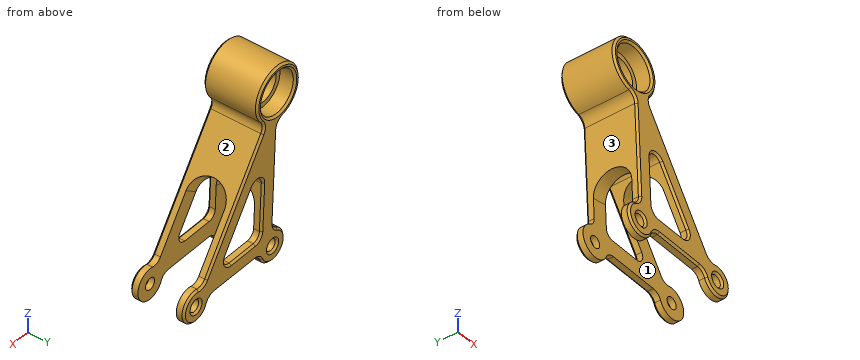
from build123d import *

# Parameters (mm, degrees)
SKETCH1_R                       = 14
BOSS_EXTRUDE1_DEPTH             = 14
SKETCH4_R                       = 11
CUT_EXTRUDE1_DEPTH              = 8
SKETCH5_R                       = 8.5
CUT_EXTRUDE2_DEPTH              = 21
BOSS_EXTRUDE2_REACH             = 16
BOSS_EXTRUDE2_DIRECTION_2_REACH = 16
SKETCH8_R                       = 3
CUT_EXTRUDE3_DEPTH              = 15
CUT_EXTRUDE3_DEPTH_BACK         = 15
FILLET1_R                       = 5
FILLET2_R                       = 4
CHAMFER1_SIZE                   = 1


with BuildPart() as part:
    # Sketch1 → Boss-Extrude1 (new body, symmetric)
    with BuildSketch(Plane(origin=(0, 0, 0), x_dir=(1, 0, 0), z_dir=(0, 1, 0))):
        Circle(SKETCH1_R)
    extrude(amount=BOSS_EXTRUDE1_DEPTH, both=True)

    # Sketch4 → Cut-Extrude1 (cut)
    with BuildSketch(Plane(origin=(0, 14, 0), x_dir=(1, 0, 0), z_dir=(0, 1, 0))):
        Circle(SKETCH4_R)
    cut_extrude1 = extrude(amount=-CUT_EXTRUDE1_DEPTH, mode=Mode.SUBTRACT)

    # Mirror1: Cut-Extrude1 across plane
    add(cut_extrude1.mirror(Plane.ZX), mode=Mode.SUBTRACT)

    # Sketch5 → Cut-Extrude2 (cut, through all)
    with BuildSketch(Plane(origin=(0, 6, 0), x_dir=(1, 0, 0), z_dir=(0, 1, 0))):
        Circle(SKETCH5_R)
    extrude(amount=-CUT_EXTRUDE2_DEPTH, mode=Mode.SUBTRACT)

    # Boss-Extrude2: up to this face of the body (flat: up to its plane)
    boss_extrude2_end = Plane(part.part.faces().sort_by_distance((-13.604020203, 14, 0))[0])
    # Sketch6 → Boss-Extrude2 (add, up to the picked face)
    with BuildSketch(Plane(origin=(0, 0, 0), x_dir=(1, 0, 0), z_dir=(0, 1, 0)), mode=Mode.PRIVATE) as boss_extrude2_sk1:
        with BuildLine():
            Line((0, 0), (49.796956955, 71.339071188))
            ThreePointArc((49.796956955, 71.339071188), (61.469373279, 81.598158377), (46.37598748, 77.89898578))
            Line((46.37598748, 77.89898578), (11.968376795, 77.89898578))
            ThreePointArc((11.968376795, 77.89898578), (-1.542698235, 83.697955691), (3.56136379, 69.909346213))
            Line((3.56136379, 69.909346213), (0, 0))
        make_face()
        Polygon((9.409062598, 27.456171423), (39.035506627, 69.89898578), (11.57120987, 69.89898578), align=None, mode=Mode.SUBTRACT)
    boss_extrude2_tool1 = split(extrude(boss_extrude2_sk1.sketch, amount=BOSS_EXTRUDE2_REACH, mode=Mode.PRIVATE), bisect_by=boss_extrude2_end, keep=Keep.BOTH, mode=Mode.PRIVATE)
    add(boss_extrude2_tool1.solids().sort_by_distance((2.865029, 0, -34.899434))[0])

    # Boss-Extrude2 direction 2: up to this face of the body (flat: up to its plane)
    boss_extrude2_direction_2_end = Plane(part.part.faces().sort_by_distance((-13.604020203, -14, 0))[0])
    # Sketch6 → Boss-Extrude2 direction 2 (add, up to the picked face)
    with BuildSketch(Plane(origin=(0, 0, 0), x_dir=(1, 0, 0), z_dir=(0, 1, 0)), mode=Mode.PRIVATE) as boss_extrude2_direction_2_sk1:
        with BuildLine():
            Line((0, 0), (49.796956955, 71.339071188))
            ThreePointArc((49.796956955, 71.339071188), (61.469373279, 81.598158377), (46.37598748, 77.89898578))
            Line((46.37598748, 77.89898578), (11.968376795, 77.89898578))
            ThreePointArc((11.968376795, 77.89898578), (-1.542698235, 83.697955691), (3.56136379, 69.909346213))
            Line((3.56136379, 69.909346213), (0, 0))
        make_face()
        Polygon((9.409062598, 27.456171423), (39.035506627, 69.89898578), (11.57120987, 69.89898578), align=None, mode=Mode.SUBTRACT)
    boss_extrude2_direction_2_tool1 = split(extrude(boss_extrude2_direction_2_sk1.sketch, amount=-BOSS_EXTRUDE2_DIRECTION_2_REACH, mode=Mode.PRIVATE), bisect_by=boss_extrude2_direction_2_end, keep=Keep.BOTH, mode=Mode.PRIVATE)
    add(boss_extrude2_direction_2_tool1.solids().sort_by_distance((2.865029, 0, -34.899434))[0])

    # Sketch7 → Cut-Revolve1 (revolve, cut)
    with BuildSketch(Plane.XY):
        Polygon((0, 14), (0, -14), (11, -14), (11, -6), (8.5, -6), (8.5, 6), (11, 6), (11, 14), align=None)
    revolve(axis=Axis((0, 14, 0), (0, -1, 0)), mode=Mode.SUBTRACT)

    # Sketch8 → Cut-Extrude3 (cut, two sides)
    with BuildSketch(Plane(origin=(0, 0, 0), x_dir=(1, 0, 0), z_dir=(0, 1, 0))) as cut_extrude3_sk:
        with Locations((3.968376795, 77.89898578)):
            Circle(SKETCH8_R)
        with Locations((54.37598748, 77.89898578)):
            Circle(SKETCH8_R)
    extrude(amount=CUT_EXTRUDE3_DEPTH, mode=Mode.SUBTRACT)
    extrude(cut_extrude3_sk.sketch, amount=-CUT_EXTRUDE3_DEPTH_BACK, mode=Mode.SUBTRACT)

    # Fillet1
    fillet1_edges = [part.edges().sort_by_distance(p)[0] for p in [
        (8.013303418, 0, -11.479850536),
        (0.712272758, 0, -13.981869243),
        (3.56136379, 0, -69.909346213),
        (11.968376795, 0, -77.89898578),
        (46.37598748, 0, -77.89898578),
        (49.796956955, 0, -71.339071188),
    ]]
    fillet(fillet1_edges, radius=FILLET1_R)

    # Fillet2
    fillet2_edges = [part.edges().sort_by_distance(p)[0] for p in [
        (11.57120987, 0, -69.89898578),
        (39.035506627, 0, -69.89898578),
        (9.409062598, 0, -27.456171423),
    ]]
    fillet(fillet2_edges, radius=FILLET2_R)

    # Sketch10 → Cut-Revolve2 (revolve, cut)
    with BuildSketch(Plane.ZY.offset(4.031623205)):
        with BuildLine():
            Line((-115.89898578, 10), (-55.89898578, 10))
            ThreePointArc((-55.89898578, 10), (-45.89898578, 0), (-55.89898578, -10))
            Line((-55.89898578, -10), (-115.89898578, -10))
            Line((-115.89898578, -10), (-115.89898578, 10))
        make_face()
    revolve(axis=Axis((-4.031623205, 14, 0.161756304), (0, -1, 0)), mode=Mode.SUBTRACT)

    # Chamfer1
    chamfer1_edges = [part.edges().sort_by_distance(p)[0] for p in [
        (45.149488461, -14, -78.738734309),
        (45.149488461, 14, -78.738734309),
        (13.194875814, -14, -78.738734309),
        (13.194875814, 14, -78.738734309),
        (26.019387345, 14, -51.252106195),
        (26.019387345, -14, -51.252106195),
        (23.368946304, 14, -69.89898578),
        (23.368946304, -14, -69.89898578),
        (10.748290369, 14, -53.74512796),
        (10.748290369, -14, -53.74512796),
        (34.9119591, -14, -67.748572079),
        (34.9119591, 14, -67.748572079),
        (12.617088893, -14, -68.798470735),
        (12.617088893, 14, -68.798470735),
        (12.81684933, -14, -37.400283889),
        (12.81684933, 14, -37.400283889),
        (-6.296166971, -14, 9.019882564),
        (-6.296166971, 14, 9.019882564),
        (0.968376795, -14, -77.89898578),
        (0.968376795, 14, -77.89898578),
        (51.37598748, -14, -77.89898578),
        (51.37598748, 14, -77.89898578),
        (28.999659343, 14, -41.544883239),
        (28.999659343, -14, -41.544883239),
        (-4.538605987, 14, 13.243906361),
        (-4.538605987, -14, 13.243906361),
        (2.14522062, -14, -42.110545238),
        (2.14522062, 14, -42.110545238),
        (-1.542698235, 14, -83.697955691),
        (-1.542698235, -14, -83.697955691),
        (61.469373279, 14, -81.598158377),
        (61.469373279, -14, -81.598158377),
        (29.172182137, 14, -77.89898578),
        (29.172182137, -14, -77.89898578),
        (9.596412617, -14, -11.95458808),
        (9.596412617, 14, -11.95458808),
        (-0.246894433, 14, -15.32782941),
        (-0.246894433, -14, -15.32782941),
        (2.66030265, -14, -68.727159148),
        (2.66030265, 14, -68.727159148),
        (49.783519727, -14, -69.852700819),
        (49.783519727, 14, -69.852700819),
    ]]
    chamfer(chamfer1_edges, length=CHAMFER1_SIZE)


solid = part.part
For this review, take the finished solid that the model builds, in its own axes (mm). Face numbers are marked on the shaded views. Coordinates: 2 decimals unless noted, no trailing zeros. Loops run counter-clockwise (first coordinate to the right, second up) from the corner with the lowest first, then second, coordinate; pieces in that order, holes last. Notation, with made-up numbers: (82, 74.25) - (130, 74.25) arc R5 cw to (130, 78.25) - close; hole circle Ø1 at (15, -36). An arc over 180 degrees is marked (long way). Use a Markdown table: item, result. Add a question column.
Item 1: We need section A-A (z = 0). Give the boundary of the cut face in (x, y), and give its area (3 significant figures).
Item 2: We need section C-C (z = -59.5). Give the boundary of the cut face in (x, y).
Item 3: We need section B-B (y = -3.75). Give the boundary of the cut face in (x, z).
Item 4: Mouldability with a two-part tool opening along Z and no side actions: class the marked faces 1, 2 and 3 as pulls with the +Z half, pulls with the -Z half, needs draft (parallel to the pull), parting line crosses it, or undercut.
Item 5: We need section D-D (y = 1). Give the boundary of the cut face in (x, z), and give its area (3 significant figures).
Item 6: For line 1 (Y direction, x = 23, z = -73); line 2 (X direction, y = 2.25, z = 0); line 3 (X direction, y = -11, z = -75.5), list the stretches that pass through material, from the lowest coordinate up.
Item 7: Insertion check: pin 1 Ø2.5 at (x, y) = (22.5, -11.5) entering from +Z; pin 2 Ø2.5 at (x, y) = (29.5, 11.5) entering from -Z; pin 3 Ø1.5 at (y, z) = (9.5, -5) entering from -X. Each pin has a flat end and moves straight along its axis. Give the tip position at first contact, or say it passes through.
Results list:
| question | item | result |
|---|---|---|
| 1 | outline | (-14, -13) - (-13, -14) - (-12, -14) - (-11, -13) - (-11, -6) - (-8.5, -6) - (-8.5, 6) - (-11, 6) - (-11, 13) - (-12, 14) - (-13, 14) - (-14, 13) - close; (8.5, -6) - (11, -6) - (11, -13) - (12, -14) - (13, -14) - (14, -13) - (14, 13) - (13, 14) - (12, 14) - (11, 13) - (11, 6) - (8.5, 6) - close |
| 1 | area | 224 mm^2 |
| 2 | outline | (3.03, -13) - (4.03, -14) - (10.04, -14) - (11.04, -13) - (11.04, -10) - (3.03, -10) - close; (3.03, 10) - (11.04, 10) - (11.04, 13) - (10.04, 14) - (4.03, 14) - (3.03, 13) - close; (31.78, -13) - (33, -14) - (40.31, -14) - (41.53, -13) - (41.53, -10) - (31.78, -10) - close; (31.78, 10) - (41.53, 10) - (41.53, 13) - (40.31, 14) - (33, 14) - (31.78, 13) - close |
| 3 | outline | (-2.99, -13.68) arc R5 cw to (0.93, -18.31) - (2.35, -46.19) arc R46.79 ccw to (10.27, -44.39) - (10.12, -41.39) arc R4 cw to (17.39, -38.89) - (18.68, -40.74) arc R46.79 ccw to (25.32, -36.28) - (10.49, -15.03) arc R5 cw to (10.75, -8.97) arc R14 ccw (long way) to start; hole circle Ø17 at (0, 0) |
| 4 | face 1 | needs draft |
| 4 | face 2 | undercut |
| 4 | face 3 | undercut |
| 5 | outline | (-2.99, -13.68) arc R5 cw to (0.93, -18.31) - (2.32, -45.51) arc R46.11 ccw to (10.24, -43.69) - (10.12, -41.39) arc R4 cw to (17.39, -38.89) - (18.29, -40.18) arc R46.11 ccw to (24.93, -35.72) - (10.49, -15.03) arc R5 cw to (10.75, -8.97) arc R14 ccw (long way) to start; hole circle Ø17 at (0, 0) |
| 5 | area | 862 mm^2 |
| 6 | line 1 | y = -14 to -10, 10 to 14 |
| 6 | line 2 | x = -14 to -8.5, 8.5 to 14 |
| 6 | line 3 | x = -3.66 to 2.17, 5.77 to 52.57, 56.18 to 62.01 |
| 7 | pin 1 | stops at z = -30.44 |
| 7 | pin 2 | stops at z = -77.9 |
| 7 | pin 3 | stops at x = -13.34 |
